Design review of the part shown in the three views and the two pictorial views. Dimensions are in mm from the part's minimum x, y and z. A direction names the side the tool comes from. Give positions to 0.01 mm unless a question says otherwise; leave off trailing zeros. Loops run counter-clockwise (first coordinate to the right, second up) from the corner with the lowest first, then second, coordinate; pieces in that order, holes last. Notation, with made-up numbers: (30, 6.5) - (75, 6.5) arc R21 ccw to (75, 36.5) - close; hole circle Ø2 at (79.5, 12). An arc over 180 degrees is marked (long way). Return JSON: item names as keys, results as strings. Group by question number.
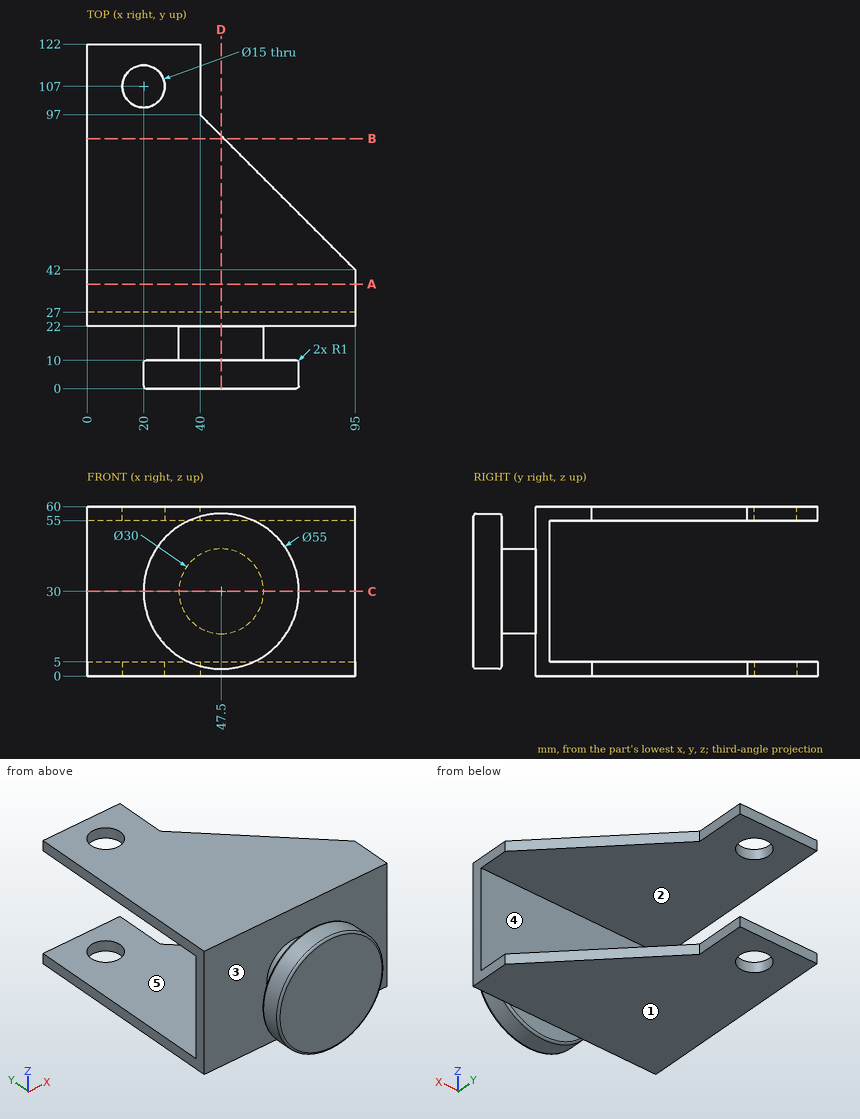
Item 1: Take a section at D-D (x = 47.5). State the section outline as (y, z) points.
Item 2: Tool access review of the marked faces 1 and 2: name each direction out of +Z, -Z, +X, -X, +Y, -Y from which nothing blocks a thin tool from reaching the whole face with its end or side.
Item 3: For L1, parallel to Y at x = 20, z = 57; L2, parallel to Y at x = 38, z = 47.5; L3, parallel to Z at x = 6.5, y = 97, list the stretches that pass through material, from the lowest coordinate up. Write a range as from..to.
Item 4: Take a section at A-A (y = 37). State the section outline as (x, z) points, then the cut area to 3 significant figures.
Item 5: Mouldability with a two-part tool opening along Y and no side actions: class the marked faces 3, 4 and 5 as +Y half, -Y half, draft (parallel to the pull), parting line (faces both ways), or undercut.
Item 6: Take a section at B-B (y = 88.5). State the section outline as (x, z) points.
Item 7: For P1, Ø4, axis at x = 12, z = 16, coming from the -Y side; P2, Ø5.5, axis at y = 109, z = 2, coming from the +X side; P3, Ø1.5, axis at x = 53.5, z = 43, coming from the +Y side, all flat-tipped, find the tip position at first contact; note any pin that passes through.
Item 8: Take a section at C-C (z = 30). State the section outline as (x, y) points, then the cut area to 3 significant figures.
Check sheet entries:
{
 "1": {"outline": "(0, 3.5) arc R1 ccw to (1, 2.5) - (9, 2.5) arc R1 ccw to (10, 3.5) - (10, 15) - (22, 15) - (22, 0) - (89.5, 0) - (89.5, 5) - (27, 5) - (27, 55) - (89.5, 55) - (89.5, 60) - (22, 60) - (22, 45) - (10, 45) - (10, 56.5) arc R1 ccw to (9, 57.5) - (1, 57.5) arc R1 ccw to (0, 56.5) - close"},
 "2": {"face 1": "-Z, +X, -X, +Y, -Y", "face 2": "+X, -X, +Y"},
 "3": {"L1": "y = 22..99.5, 114.5..122", "L2": "y = 0..10, 22..27", "L3": "z = 0..5, 55..60"},
 "4": {"outline": "(0, 0) - (95, 0) - (95, 5) - (0, 5) - close; (0, 55) - (95, 55) - (95, 60) - (0, 60) - close", "area": "950 mm^2"},
 "5": {"face 3": "undercut", "face 4": "+Y half", "face 5": "draft"},
 "6": {"outline": "(0, 0) - (48.5, 0) - (48.5, 5) - (0, 5) - close; (0, 55) - (48.5, 55) - (48.5, 60) - (0, 60) - close"},
 "7": {"P1": "stops at y = 22", "P2": "stops at x = 40", "P3": "stops at y = 27"},
 "8": {"outline": "(0, 22) - (32.5, 22) - (32.5, 10) - (21, 10) arc R1 ccw to (20, 9) - (20, 1) arc R1 ccw to (21, 0) - (74, 0) arc R1 ccw to (75, 1) - (75, 9) arc R1 ccw to (74, 10) - (62.5, 10) - (62.5, 22) - (95, 22) - (95, 27) - (0, 27) - close", "area": "1,380 mm^2"}
}
